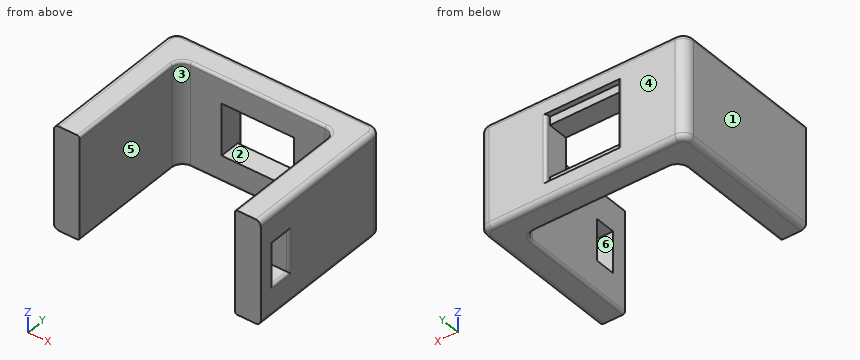
```python
from build123d import *

# Parameters (mm, degrees)
BOSS_EXTRUDE1_DEPTH = 50.8
FILLET1_R           = 5.08
SKETCH2_W           = 35.56
SKETCH2_H           = 33.528
CUT_EXTRUDE1_DEPTH  = 2.54
SKETCH4_W           = 35.56
SKETCH4_H           = 25.4
CUT_EXTRUDE2_DEPTH  = 74.66
FILLET2_R           = 1.27
CUT_EXTRUDE3_REACH  = 103.6
SKETCH6_W           = 20.32
SKETCH6_H           = 10.16
FILLET3_R           = 2.54
FILLET4_R           = 1.27
FILLET5_R           = 1.27


with BuildPart() as part:
    # Sketch1 → Boss-Extrude1 (new body)
    with BuildSketch(Plane.XY):
        Polygon((0, 0), (0, 76.2), (101.6, 76.2), (101.6, 0), (88.9, 0), (88.9, 63.5), (12.7, 63.5), (12.7, 0), align=None)
    extrude(amount=BOSS_EXTRUDE1_DEPTH)

    # Fillet1
    fillet1_edges = [part.edges().sort_by_distance(p)[0] for p in [
        (0, 76.2, 25.4),
        (101.6, 76.2, 25.4),
        (88.9, 63.5, 25.4),
        (12.7, 63.5, 25.4),
    ]]
    fillet(fillet1_edges, radius=FILLET1_R)

    # Sketch2 → Cut-Extrude1 (cut)
    with BuildSketch(Plane(origin=(0, 76.2, 0), x_dir=(1, 0, 0), z_dir=(0, 1, 0))):
        with Locations((50.8, -25.4)):
            Rectangle(SKETCH2_W, SKETCH2_H)
    extrude(amount=-CUT_EXTRUDE1_DEPTH, mode=Mode.SUBTRACT)

    # Sketch4 → Cut-Extrude2 (cut, through all)
    with BuildSketch(Plane(origin=(0, 73.66, 0), x_dir=(1, 0, 0), z_dir=(0, 1, 0))):
        with Locations((50.8, -25.4)):
            Rectangle(SKETCH4_W, SKETCH4_H)
    extrude(amount=-CUT_EXTRUDE2_DEPTH, mode=Mode.SUBTRACT)

    # Fillet2
    fillet2_edges = [part.edges().sort_by_distance(p)[0] for p in [
        (68.58, 76.2, 25.4),
        (33.02, 76.2, 25.4),
    ]]
    fillet(fillet2_edges, radius=FILLET2_R)

    # Sketch6 → Cut-Extrude3 (cut, up to next)
    with BuildSketch(Plane(origin=(101.6, 0, 0), x_dir=(0, 0, -1), z_dir=(1, 0, 0)), mode=Mode.PRIVATE) as cut_extrude3_sk1:
        with Locations((-25.4, 12.7)):
            Rectangle(SKETCH6_W, SKETCH6_H)
    cut_extrude3_tool1 = extrude(cut_extrude3_sk1.sketch, amount=-CUT_EXTRUDE3_REACH, mode=Mode.PRIVATE) & part.part
    add(cut_extrude3_tool1.solids().sort_by_distance((101.6, 12.7, 25.4))[0], mode=Mode.SUBTRACT)

    # Fillet3
    fillet3_edges = [part.edges().sort_by_distance(p)[0] for p in [
        (101.6, 35.56, 50.8),
        (50.8, 76.2, 0),
        (50.8, 76.2, 50.8),
        (0, 35.56, 0),
        (1.487897552, 74.712102448, 0),
        (100.112102448, 74.712102448, 0),
        (0, 35.56, 50.8),
        (1.487897552, 74.712102448, 50.8),
        (100.112102448, 74.712102448, 50.8),
        (101.6, 35.56, 0),
    ]]
    fillet(fillet3_edges, radius=FILLET3_R)

    # Fillet4
    fillet4_edges = [part.edges().sort_by_distance(p)[0] for p in [
        (101.6, 12.7, 35.56),
        (101.6, 17.78, 25.4),
        (101.6, 7.62, 25.4),
        (101.6, 12.7, 15.24),
    ]]
    fillet(fillet4_edges, radius=FILLET4_R)

    # Fillet5
    fillet5_edges = [part.edges().sort_by_distance(p)[0] for p in [
        (12.7, 29.21, 0),
        (88.9, 29.21, 0),
        (88.9, 29.21, 50.8),
        (50.8, 63.5, 0),
        (50.8, 63.5, 50.8),
        (87.412102448, 62.012102448, 0),
        (87.412102448, 62.012102448, 50.8),
        (14.187897552, 62.012102448, 0),
        (14.187897552, 62.012102448, 50.8),
        (12.7, 29.21, 50.8),
    ]]
    fillet(fillet5_edges, radius=FILLET5_R)


solid = part.part
```
Source: CAD feature listing. Evaluate the final solid. Frame: model axes, mm. Face numbers are marked on the shaded views. A direction names the side the tool comes from. Give positions to 0.01 mm unless a question says otherwise; leave off trailing zeros. Order: outer loops, then holes, each group sorted by start corner. A loop starts at its lowest first (then second) coordinate and runs counter-clockwise, first axis right, second up.
(1) Section query C-C (x = 37). Return the cut outline in (y, z), plus the area to 3 significant figures.
(2) Material intervals for line 1 along X through (y, z) = (53.5, 11.5); line 2 along Y through (x, z) = (91, 17); line 3 along X through (y, z) = (71, 26), sorted ascending.
(3) Section query A-A (z = 19.5). Return the cut outline in (x, y), plus the area to 3 significant figures.
(4) Pull-direction query (Y, two-part tool) for the marked faces 4, 5 and 6; classes: +Y half, -Y half, draft (parallel to the pull), parting line (faces both ways), or undercut.
(5) Section query D-D (y = 14). Return the cut outline in (x, z).
(6) Access query for the marked faces 1, 2 and 3. Directions: +Z, -Z, +X, -X, +Y, -Y. A direction counts if a zero-diameter tool reaches every point of the face in a straight line with its end or side. Return the directions, or none.
(7) Contact query for flat-ended pins moving along their axis: P1, Ø0.8, axis at x = 43, y = 75, coming from the +Z side; P2, Ø3.5, axis at x = 96.5, z = 20.5, coming from the -Y side; P3, Ø3.5, axis at x = 49.5, z = 11, coming from the +Y side. Output: stop coordinate, or through.
(8) Section query B-B (y = 52.5). Return the cut outline in (x, z), plus the area to 3 significant figures.
Outcome:
1. outline: (63.5, 1.27) arc R1.27 ccw to (64.77, 0) - (73.66, 0) arc R2.54 ccw to (76.2, 2.54) - (76.2, 8.64) - (73.66, 8.64) - (73.66, 12.7) - (63.5, 12.7) - close; (63.5, 38.1) - (73.66, 38.1) - (73.66, 42.16) - (76.2, 42.16) - (76.2, 48.26) arc R2.54 ccw to (73.66, 50.8) - (64.77, 50.8) arc R1.27 ccw to (63.5, 49.53) - close
1. area: 298 mm2
2. line 1: x = 0 to 12.7, 88.9 to 101.6
2. line 2: y = 0 to 7.62, 17.78 to 76.2
2. line 3: x = 0 to 33.02, 68.58 to 101.6
3. outline: (0, 0) - (12.7, 0) - (12.7, 58.42) arc R5.08 cw to (17.78, 63.5) - (33.02, 63.5) - (33.02, 74.93) arc R1.27 ccw to (31.75, 76.2) - (5.08, 76.2) arc R5.08 ccw to (0, 71.12) - close; (68.58, 63.5) - (83.82, 63.5) arc R5.08 cw to (88.9, 58.42) - (88.9, 17.78) - (100.33, 17.78) arc R1.27 ccw to (101.6, 19.05) - (101.6, 71.12) arc R5.08 ccw to (96.52, 76.2) - (69.85, 76.2) arc R1.27 ccw to (68.58, 74.93) - close; (88.9, 0) - (101.6, 0) - (101.6, 6.35) arc R1.27 ccw to (100.33, 7.62) - (88.9, 7.62) - close
3. area: 2,320 mm2
4. face 4: +Y half
4. face 5: draft
4. face 6: undercut
5. outline: (0, 2.54) arc R2.54 ccw to (2.54, 0) - (11.43, 0) arc R1.27 ccw to (12.7, 1.27) - (12.7, 49.53) arc R1.27 ccw to (11.43, 50.8) - (2.54, 50.8) arc R2.54 ccw to (0, 48.26) - close; (88.9, 1.27) arc R1.27 ccw to (90.17, 0) - (99.06, 0) arc R2.54 ccw to (101.6, 2.54) - (101.6, 13.97) arc R1.27 ccw to (100.33, 15.24) - (88.9, 15.24) - close; (88.9, 35.56) - (100.33, 35.56) arc R1.27 ccw to (101.6, 36.83) - (101.6, 48.26) arc R2.54 ccw to (99.06, 50.8) - (90.17, 50.8) arc R1.27 ccw to (88.9, 49.53) - close
6. face 1: +Z, -Z, -X, +Y, -Y
6. face 2: +Y, -Y
6. face 3: +Z, -Z, -Y
7. P1: stops at z = 50.62
7. P2: stops at y = 0
7. P3: stops at y = 73.66
8. outline: (0, 2.54) arc R2.54 ccw to (2.54, 0) - (11.43, 0) arc R1.27 ccw to (12.7, 1.27) - (12.7, 49.53) arc R1.27 ccw to (11.43, 50.8) - (2.54, 50.8) arc R2.54 ccw to (0, 48.26) - close; (88.9, 1.27) arc R1.27 ccw to (90.17, 0) - (99.06, 0) arc R2.54 ccw to (101.6, 2.54) - (101.6, 48.26) arc R2.54 ccw to (99.06, 50.8) - (90.17, 50.8) arc R1.27 ccw to (88.9, 49.53) - close
8. area: 1,280 mm2
